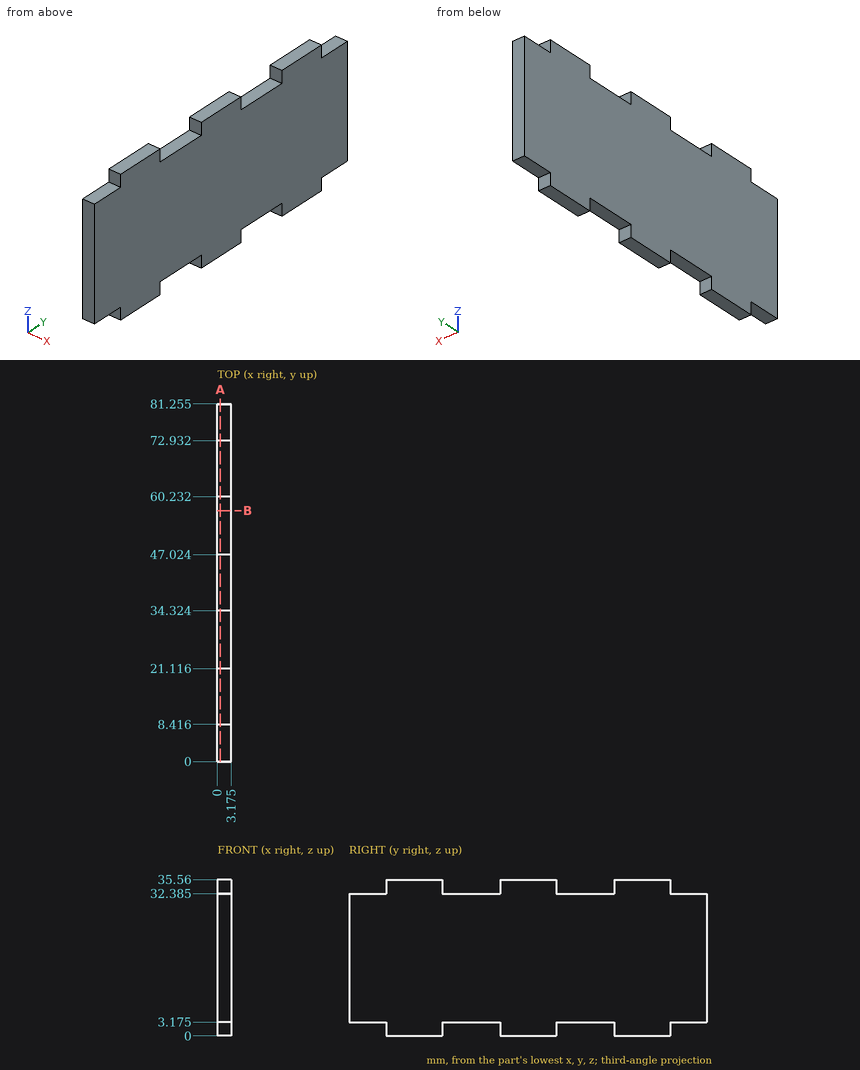
Geometry check sheet. Reference: drawing and pictorial views, mm from the part's lowest x, y, z. Round coordinates to 2 decimals unless told otherwise and drop trailing zeros. Loops run counter-clockwise (first coordinate to the right, second up) from the corner with the lowest first, then second, coordinate; pieces in that order, holes last. Notation, with made-up numbers: (47, -11) -> (56, -11) arc R18 ccw to (56, -5) -> close; hole circle Ø3 at (20.25, 46.5). An arc over 180 degrees is marked (long way). Answer as a JSON object with one key per item and string values.
Q1. Section check A-A (x = 0.7). Record the boundary of the cut face in (y, z) (1 decimal).
Data:
{"outline": "(0, 3.2) -> (8.4, 3.2) -> (8.4, 0) -> (21.1, 0) -> (21.1, 3.2) -> (34.3, 3.2) -> (34.3, 0) -> (47, 0) -> (47, 3.2) -> (60.2, 3.2) -> (60.2, 0) -> (72.9, 0) -> (72.9, 3.2) -> (81.3, 3.2) -> (81.3, 32.4) -> (72.9, 32.4) -> (72.9, 35.6) -> (60.2, 35.6) -> (60.2, 32.4) -> (47, 32.4) -> (47, 35.6) -> (34.3, 35.6) -> (34.3, 32.4) -> (21.1, 32.4) -> (21.1, 35.6) -> (8.4, 35.6) -> (8.4, 32.4) -> (0, 32.4) -> close"}
Q2. Scan line: line 1 (Z direction, x = 0.7, y = 56.5) (1 decimal). Record every from-to range of solid material in increasing order. Write a range as from..to.
Data:
{"line 1": "z = 3.2..32.4"}
Q3. Go/stop test with flat-tipped pins: P1, Ø1, axis at x = 2.5, z = 2, coming from the -Y side; P2, Ø1.6, axis at x = 2, y = 79, coming from the -Z side (3 decimals); P3, Ø1.6, axis at x = 1.5, y = 26, coming from the +Z side (3 decimals). Record where each tip stops, or that it passes through.
Data:
{"P1": "stops at y = 8.42", "P2": "stops at z = 3.175", "P3": "stops at z = 32.385"}
Q4. Section check B-B (y = 57). Record the boundary of the cut face in (x, z) (1 decimal).
Data:
{"outline": "(0, 3.2) -> (3.2, 3.2) -> (3.2, 32.4) -> (0, 32.4) -> close"}
